Design review of the part built by this model. Coordinates are the model's own, in mm. A direction names the side the tool comes from. Coordinates: 2 decimals unless noted, no trailing zeros. Loops run counter-clockwise (first coordinate to the right, second up) from the corner with the lowest first, then second, coordinate; pieces in that order, holes last. Notation, with made-up numbers: (44, -0.75) -> (87, -0.75) arc R35 cw to (87, 36.25) -> close; hole circle Ø8 at (5, 6.5). An arc over 180 degrees is marked (long way). Use one line per item in the form item = value. Start each with the question number.
1. The part is to be moulded in two halves that separate along Y. For faces 1 (the face through (-44.602, -35, 1)), 2 (the face through (-39.602, -57, 1)), 3 (the face through (-60, -26, 1)), say which applies: released by +Y, released by -Y, zero draft, split by the parting line, or undercut.
2. Machinability: for faces 4 (the face through (-61, -88, 1)), 5 (the face through (-76.602, -35, 1)), which of the approach directions +Z, -Z, +X, -X, +Y, -Y give a long, thin tool a straight path to every point of the face, cutting with its end or side? Answer none if there is none.
3. Consider section D-D (z = 1.65). State the section outline as (x, y) points.
4. Consider section A-A (x = -64). State the section outline as (y, z) points, then the cut area to 3 significant figures.
5. Consider section C-C (y = -42). State the section outline as (x, z) points, then the cut area to 3 significant figures.
6. For pin 1 (1.8 mm diameter, centred on x = -48.1, y = -79.5, fed in from +Z), flat-tipped, find the tip position at first contact; note if it passes through.
7. Wall thickness on line 1 (Y direction, x = -54, z = 0.2); line 2 (X direction, y = -65, z = 0.25); line 3 (Y direction, x = -50, z = 0.2): over which ranges is each line inside the solid? List them lowest first. Write a range as from..to.
8. Consider section B-B (y = -48.5). State the section outline as (x, z) points, then the cut area to 3 significant figures.
from build123d import *

# Parameters (mm, degrees)
SKETCH1_R           = 3.5
SKETCH1_R_2         = 1.5
BOSS_EXTRUDE1_DEPTH = 2


with BuildPart() as part:
    # Sketch1 → Boss-Extrude1 (new body)
    with BuildSketch(Plane.XY):
        with BuildLine():
            ThreePointArc((-73.101516296, -83), (-75.576390016, -81.974873749), (-76.601516296, -79.500000041))
            Line((-76.601516296, -79.500000041), (-76.601516296, -83))
            Line((-76.601516296, -83), (-73.101516296, -83))
        make_face()
        with Locations((-73.101516296, -79.5)):
            Circle(SKETCH1_R)
        with Locations((-73.101516296, -79.5)):
            Circle(SKETCH1_R_2, mode=Mode.SUBTRACT)
        with BuildLine():
            Line((-44.601516296, -83), (-44.601516296, -79.5))
            ThreePointArc((-44.601516296, -79.5), (-45.626642562, -81.974873734), (-48.101516296, -83))
            Line((-48.101516296, -83), (-44.601516296, -83))
        make_face()
        with Locations((-48.101516296, -79.5)):
            Circle(SKETCH1_R)
        with Locations((-48.101516296, -79.5)):
            Circle(SKETCH1_R_2, mode=Mode.SUBTRACT)
        with BuildLine():
            ThreePointArc((-76.601516296, -50.477288358), (-79.44300278, -53.809155179), (-81.601516296, -57.61916848))
            Line((-81.601516296, -57.61916848), (-81.601516296, -76.38083152))
            ThreePointArc((-81.601516296, -76.38083152), (-76.864972263, -83.263455967), (-69.982347816, -88))
            Line((-69.982347816, -88), (-51.220684776, -88))
            ThreePointArc((-51.220684776, -88), (-44.338060329, -83.263455967), (-39.601516296, -76.38083152))
            Line((-39.601516296, -76.38083152), (-39.601516296, -57.61916848))
            ThreePointArc((-39.601516296, -57.61916848), (-41.760029812, -53.809155179), (-44.601516296, -50.477288358))
            Line((-44.601516296, -50.477288358), (-44.601516296, -79.5))
            Line((-44.601516296, -79.5), (-44.601516296, -83))
            Line((-44.601516296, -83), (-48.101516296, -83))
            Line((-48.101516296, -83), (-73.101516296, -83))
            Line((-73.101516296, -83), (-76.601516296, -83))
            Line((-76.601516296, -83), (-76.601516296, -79.500000041))
            Line((-76.601516296, -79.500000041), (-76.601516296, -50.477288358))
        make_face()
        with BuildLine():
            ThreePointArc((-69.982347816, -88), (-76.864972263, -83.263455967), (-81.601516296, -76.38083152))
            Line((-81.601516296, -76.38083152), (-81.601516296, -88))
            Line((-81.601516296, -88), (-69.982347816, -88))
        make_face()
        with BuildLine():
            Line((-39.601516296, -88), (-39.601516296, -76.38083152))
            ThreePointArc((-39.601516296, -76.38083152), (-44.338060329, -83.263455967), (-51.220684776, -88))
            Line((-51.220684776, -88), (-39.601516296, -88))
        make_face()
        with BuildLine():
            Line((-39.601516296, -26), (-81.601516296, -26))
            Line((-81.601516296, -26), (-81.601516296, -57.61916848))
            ThreePointArc((-81.601516296, -57.61916848), (-79.44300278, -53.809155179), (-76.601516296, -50.477288358))
            Line((-76.601516296, -50.477288358), (-76.601516296, -45.354101966))
            ThreePointArc((-76.601516296, -45.354101966), (-74.101516296, -42), (-76.601516296, -38.645898034))
            Line((-76.601516296, -38.645898034), (-76.601516296, -31))
            Line((-76.601516296, -31), (-44.601516296, -31))
            Line((-44.601516296, -31), (-44.601516296, -38.645898034))
            ThreePointArc((-44.601516296, -38.645898034), (-47.101516296, -42), (-44.601516296, -45.354101966))
            Line((-44.601516296, -45.354101966), (-44.601516296, -50.477288358))
            ThreePointArc((-44.601516296, -50.477288358), (-41.760029812, -53.809155179), (-39.601516296, -57.61916848))
            Line((-39.601516296, -57.61916848), (-39.601516296, -26))
        make_face()
        with Locations((-77.601516296, -42)):
            Circle(SKETCH1_R_2, mode=Mode.SUBTRACT)
        with Locations((-43.601516296, -42)):
            Circle(SKETCH1_R_2, mode=Mode.SUBTRACT)
    extrude(amount=BOSS_EXTRUDE1_DEPTH)


solid = part.part
Geometry check:
q1.face_1 = undercut
q1.face_2 = zero draft
q1.face_3 = released by +Y
q2.face_4 = +Z, -Z, +X, -X, -Y
q2.face_5 = +Z, -Z
q3.outline = (-81.6, -88) -> (-39.6, -88) -> (-39.6, -26) -> (-81.6, -26) -> close; hole circle Ø3 at (-77.6, -42); hole (-76.6, -79.5) arc R3.5 cw (long way) to (-73.1, -83) -> (-48.1, -83) arc R3.5 cw (long way) to (-44.6, -79.5) -> (-44.6, -45.35) arc R3.5 cw to (-44.6, -38.65) -> (-44.6, -31) -> (-76.6, -31) -> (-76.6, -38.65) arc R3.5 cw to (-76.6, -45.35) -> close; hole circle Ø3 at (-73.1, -79.5); hole circle Ø3 at (-48.1, -79.5); hole circle Ø3 at (-43.6, -42)
q4.outline = (-88, 0) -> (-83, 0) -> (-83, 2) -> (-88, 2) -> close; (-31, 0) -> (-26, 0) -> (-26, 2) -> (-31, 2) -> close
q4.area = 20.0 mm²
q5.outline = (-81.6, 0) -> (-79.1, 0) -> (-79.1, 2) -> (-81.6, 2) -> close; (-76.1, 0) -> (-74.1, 0) -> (-74.1, 2) -> (-76.1, 2) -> close; (-47.1, 0) -> (-45.1, 0) -> (-45.1, 2) -> (-47.1, 2) -> close; (-42.1, 0) -> (-39.6, 0) -> (-39.6, 2) -> (-42.1, 2) -> close
q5.area = 18.0 mm²
q6.pin_1 = through
q7.line_1 = -88..-83, -31..-26
q7.line_2 = -81.6..-76.6, -44.6..-39.6
q7.line_3 = -88..-83, -82.44..-76.56, -31..-26
q8.outline = (-81.6, 0) -> (-76.6, 0) -> (-76.6, 2) -> (-81.6, 2) -> close; (-44.6, 0) -> (-39.6, 0) -> (-39.6, 2) -> (-44.6, 2) -> close
q8.area = 20.0 mm²
